Could you check a few things on this drawing? It's one solid part, dimensions in mm from its lowest x, y, z. A direction names the side the tool comes from. Give positions to 0.01 mm unless a question says otherwise; leave off trailing zeros. Order: outer loops, then holes, each group sorted by start corner. A loop starts at its lowest first (then second) coordinate and runs counter-clockwise, first axis right, second up. Notation, with made-up numbers: M 19.25,-23.75 L 25.25,-23.75 A8 ccw 25.25,-17.75 Z; hole C -1,10.25 d5. An arc over 180 degrees is marked long. One line per item, written item: value. Start each with the question number.
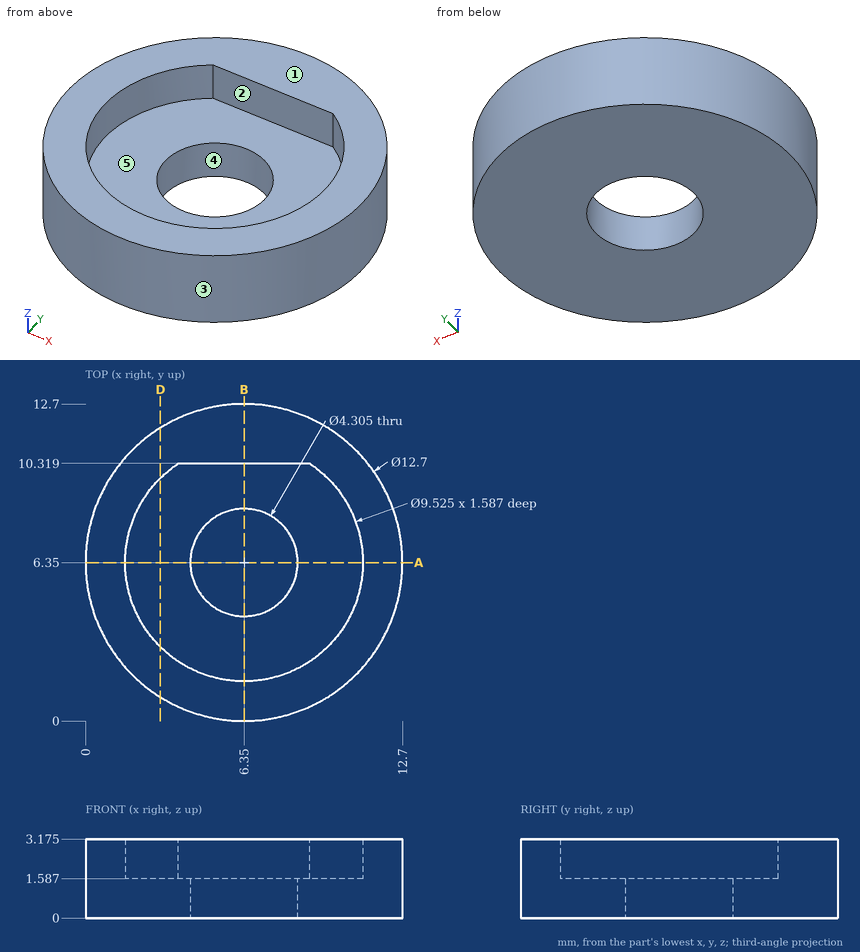
Item 1: I want a section at A-A on y = 6.35. Write out the boundary of the cut face in (x, z) (1 decimal).
Item 2: Will these pins go through, and if not, where does the flat tip stop? P1, Ø0.8, axis at x = 7.5, z = 2.5, coming from the -Y side (1 decimal); P2, Ø1, axis at x = 11, z = 1.5, coming from the -Y side (1 decimal); P3, Ø7, axis at x = 6.35, y = 6.35, coming from the +Z side.
Item 3: For the marked faces 4 and 5, which set-ups out of +Z, -Z, +X, -X, +Y, -Y let a thin tool reach every point of the face, with its end or its side?
Item 4: I want a section at B-B on x = 6.35. Write out the boundary of the cut face in (y, z) (1 decimal).
Item 5: We'd pull the mould along Y, two halves only. Please class the marked faces 1, 2 and 3: +Y half, -Y half, draft (parallel to the pull), parting line (faces both ways), or undercut.
Item 6: I want a section at D-D on x = 3. Write out the boundary of the cut face in (y, z) (1 decimal).
Item 7: Please list where these lines run through material, in increasing order: probe 1 along Y at (x, z) = (6.35, 2.85); probe 2 along Y at (x, z) = (6.35, 0.7); probe 3 along Z at (x, y) = (5, 9.25). Write a range as [from, to].
Answer below:
1. outline: M 0,0 L 4.2,0 L 4.2,1.6 L 1.6,1.6 L 1.6,3.2 L 0,3.2 Z; M 8.5,0 L 12.7,0 L 12.7,3.2 L 11.1,3.2 L 11.1,1.6 L 8.5,1.6 Z
2. P1: stops at y = 0
2. P2: stops at y = 1.5
2. P3: stops at z = 1.59
3. face 4: +Z, -Z
3. face 5: +Z
4. outline: M 0,0 L 4.2,0 L 4.2,1.6 L 1.6,1.6 L 1.6,3.2 L 0,3.2 Z; M 8.5,0 L 12.7,0 L 12.7,3.2 L 10.3,3.2 L 10.3,1.6 L 8.5,1.6 Z
5. face 1: draft
5. face 2: undercut
5. face 3: parting line
6. outline: M 1,0 L 11.7,0 L 11.7,3.2 L 9.7,3.2 L 9.7,1.6 L 3,1.6 L 3,3.2 L 1,3.2 Z
7. probe 1: y = [0, 1.59], [10.32, 12.7]
7. probe 2: y = [0, 4.2], [8.5, 12.7]
7. probe 3: z = [0, 1.59]
